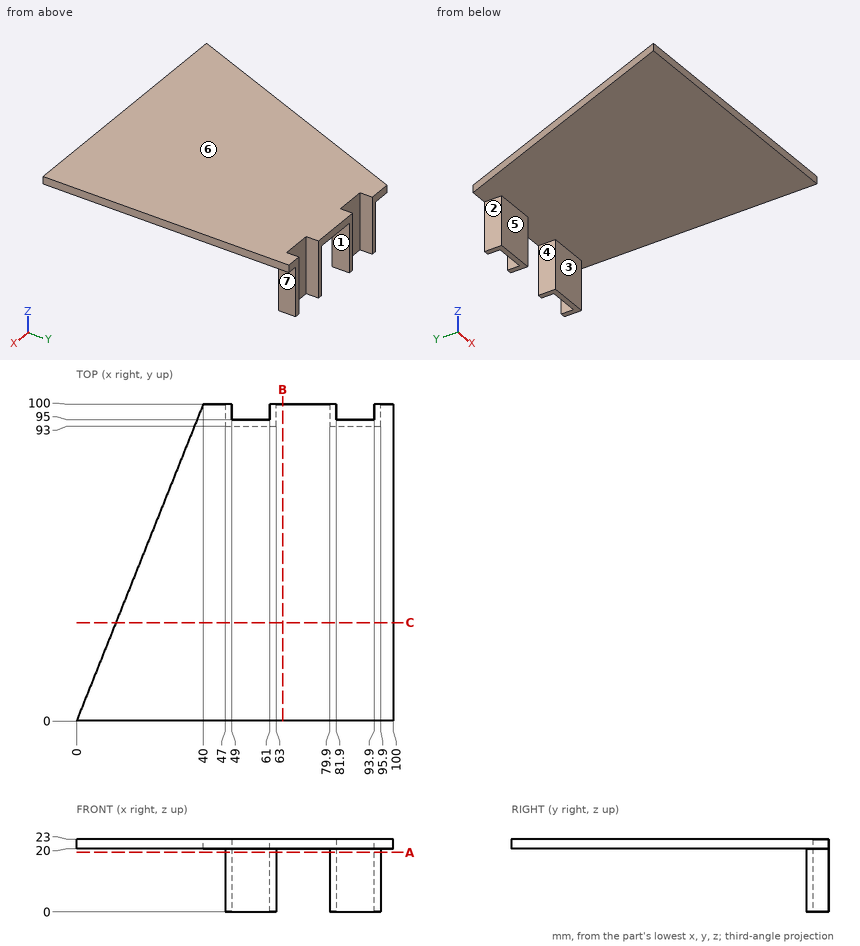
Geometry: see drawing. Coordinates: mm, zero at the bounding-box minimum. A direction names the side the tool comes from. Coordinates: 2 decimals unless noted, no trailing zeros. Write each loop counter-clockwise with the first axis right and the second up, starting at its lowest first coordinate (ties: lowest second). Pieces come first, ordered by that corner, then holes.
1) Section C-C on y = 31. Output: boundary loops of the cut face in (x, z), and give its area (3 significant figures).
2) Section B-B on x = 65. Output: boundary loops of the cut face in (y, z).
3) Mould query, pull axis X, two halves, no side actions, for the marked faces 1, 2, 3 and 4. Classes: pulls with the +X half, pulls with the -X half, needs draft (parallel to the pull), parting line crosses it, or undercut.
4) Pin query (flat end, axial travel): pin 1 Ø5.5 at (y, z) = (96.5, 12) entering from +X; pin 2 Ø6 at (x, z) = (54.5, 7.5) entering from +Y; pin 3 Ø4 at (y, z) = (97, 14) entering from -X. Return the tip coordinate at first contact, or that it passes through.
5) Set-up query: the marked faces 5, 6 and 7. Return all of +Z, -Z, +X, -X, +Y, -Y with unobstructed straight access to the full face (end or side cutting, diameter ignored); none if empty.
6) Section A-A on z = 18.75. Output: boundary loops of the cut face in (x, y).
7) Material intervals for line 1 along Z through (x, y) = (64.5, 29); line 2 along Y through (x, z) = (57, 12.75); line 3 along Y through (x, z) = (94, 17.5), sorted ascending.
Check result:
1. outline: (12.4, 20) - (100, 20) - (100, 23) - (12.4, 23) - close
1. area: 263 mm2
2. outline: (0, 20) - (100, 20) - (100, 23) - (0, 23) - close
3. face 1: undercut
3. face 2: pulls with the -X half
3. face 3: needs draft
3. face 4: undercut
4. pin 1: stops at x = 95.9
4. pin 2: stops at y = 95
4. pin 3: stops at x = 47
5. face 5: -Z, +X, -X, -Y
5. face 6: +Z, +X, -X, +Y, -Y
5. face 7: -Z, +X, +Y, -Y
6. outline: (47, 93) - (63, 93) - (63, 100) - (61, 100) - (61, 95) - (49, 95) - (49, 100) - (47, 100) - close; (79.9, 93) - (95.9, 93) - (95.9, 100) - (93.9, 100) - (93.9, 95) - (81.9, 95) - (81.9, 100) - (79.9, 100) - close
7. line 1: z = 20 to 23
7. line 2: y = 93 to 95
7. line 3: y = 93 to 100
